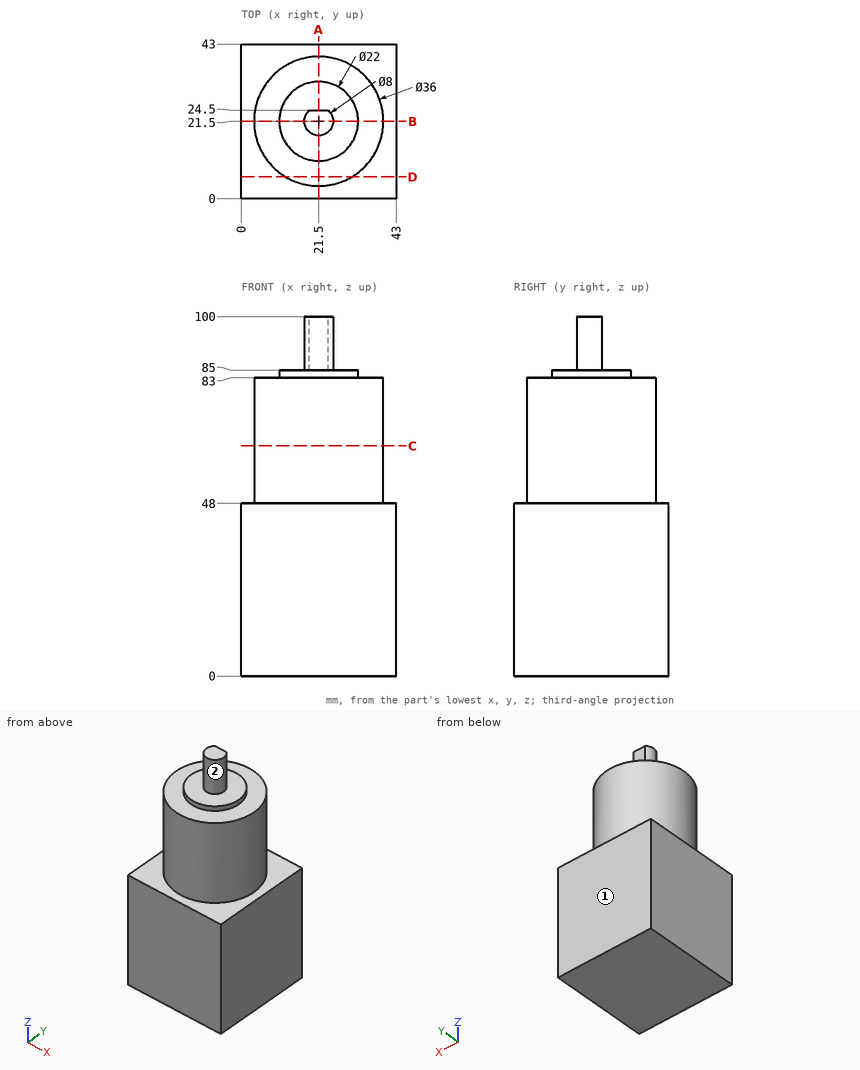
Print and shaded views of the part. All mm, measured from the part's lowest x, y and z. A direction names the side the tool comes from. Coordinates: 2 decimals unless noted, no trailing zeros. Loops run counter-clockwise (first coordinate to the right, second up) from the corner with the lowest first, then second, coordinate; pieces in that order, holes last. Notation, with made-up numbers: (18.5, 15) - (37.5, 15) arc R22 cw to (37.5, 40) - close; hole circle Ø3 at (-37.5, 38.5). An arc over 180 degrees is marked (long way). Use one line per item in the form item = value. Start each with the question number.
1) Band-saw the part on D-D (y = 6). Give the cut face in (x, z).
2) Band-saw the part on A-A (x = 21.5). Give the cut face in (y, z), and give its area (3 significant figures).
3) Flat gauge pins, fed straight in: pin 1 (8 mm diameter, centred on y = 34.5, z = 66.5, fed in from +X); pin 2 (6 mm diameter, centred on x = 21, y = 18.5, fed in from -Z); pin 3 (3 mm diameter, centred on x = 34.5, y = 10.5, fed in from +Z); pin 4 (2.5 mm diameter, centred on x = 21, z = 96, fed in from +Y). Where does each tip first touch, or does it go through?
4) Drill centre lines: L1, parallel to Z at x = 33, y = 17; L2, parallel to Z at x = 21, y = 28; L3, parallel to Y at x = 21.5, z = 65.5. Where is each one in solid material? Low to high. Write a range as from..to.
5) Band-saw the part on C-C (z = 64). Give the cut face in (x, y), and give its area (3 significant figures).
6) Tool access for the marked faces 1 and 2: list every direction of +Z, -Z, +X, -X, +Y, -Y with a clear straight run to the whole face (end or side of a thin tool).
7) Band-saw the part on B-B (y = 21.5). Give the cut face in (x, z), and give its area (3 significant figures).
Check values:
q1.outline = (0, 0) - (43, 0) - (43, 48) - (30.65, 48) - (30.65, 83) - (12.35, 83) - (12.35, 48) - (0, 48) - close
q2.outline = (0, 0) - (43, 0) - (43, 48) - (39.5, 48) - (39.5, 83) - (32.5, 83) - (32.5, 85) - (24.5, 85) - (24.5, 100) - (17.5, 100) - (17.5, 85) - (10.5, 85) - (10.5, 83) - (3.5, 83) - (3.5, 48) - (0, 48) - close
q2.area = 3,470 mm2
q3.pin_1 = 37.09
q3.pin_2 = 0
q3.pin_3 = 83
q3.pin_4 = 24.5
q4.L1 = 0..83
q4.L2 = 0..85
q4.L3 = 3.5..39.5
q5.outline = circle Ø36 at (21.5, 21.5)
q5.area = 1,020 mm2
q6.face_1 = +Z, -Z, +X, -X, +Y
q6.face_2 = +Z
q7.outline = (0, 0) - (43, 0) - (43, 48) - (39.5, 48) - (39.5, 83) - (32.5, 83) - (32.5, 85) - (25.5, 85) - (25.5, 100) - (17.5, 100) - (17.5, 85) - (10.5, 85) - (10.5, 83) - (3.5, 83) - (3.5, 48) - (0, 48) - close
q7.area = 3,490 mm2
